Geometry check sheet. Reference: the model listing, model coordinates, mm. Round coordinates to 2 decimals unless told otherwise and drop trailing zeros. Order: outer loops, then holes, each group sorted by start corner. A loop starts at its lowest first (then second) coordinate and runs counter-clockwise, first axis right, second up. Notation, with made-up numbers: (89.25, 45.5) - (129.25, 45.5) arc R29 ccw to (129.25, 70.5) - close; hole circle Ø5 at (33.5, 35). An arc over 180 degrees is marked (long way). Answer as CSV lines item,"result". Start each with the question number.
```python
from build123d import *

# Parameters (mm, degrees)
SKETCH1_W           = 228.6
SKETCH1_H           = 457.2
BOSS_EXTRUDE1_DEPTH = 6.35
SKETCH2_W           = 6.35
SKETCH2_H           = 76.2
BOSS_EXTRUDE4_DEPTH = 6.35
SKETCH3_W           = 76.2
SKETCH3_H           = 6.35
CUT_EXTRUDE1_DEPTH  = 6.35


with BuildPart() as part:
    # Sketch1 → Boss-Extrude1 (new body)
    with BuildSketch(Plane.XY):
        with Locations((-78.307659574, -48.638297872)):
            Rectangle(SKETCH1_W, SKETCH1_H)
    extrude(amount=BOSS_EXTRUDE1_DEPTH)

    # Sketch2 → Boss-Extrude4 (add, through all)
    with BuildSketch(Plane.XY.offset(6.35)):
        with Locations((-195.782659574, 59.311702128)):
            Rectangle(SKETCH2_W, SKETCH2_H)
        with Locations((-195.782659574, -156.588297872)):
            Rectangle(SKETCH2_W, SKETCH2_H)
        with Locations((39.167340426, -156.588297872)):
            Rectangle(SKETCH2_W, SKETCH2_H)
        with Locations((39.167340426, 59.311702128)):
            Rectangle(SKETCH2_W, SKETCH2_H)
    extrude(amount=-BOSS_EXTRUDE4_DEPTH)

    # Sketch3 → Cut-Extrude1 (cut)
    with BuildSketch(Plane.XY.offset(6.35)):
        with Locations((-129.107659574, -274.063297872)):
            Rectangle(SKETCH3_W, SKETCH3_H)
        with Locations((-27.507659574, -274.063297872)):
            Rectangle(SKETCH3_W, SKETCH3_H)
        with Locations((-78.307659574, 176.786702128)):
            Rectangle(SKETCH3_W, SKETCH3_H)
    extrude(amount=-CUT_EXTRUDE1_DEPTH, mode=Mode.SUBTRACT)


solid = part.part
```
1. Thickness scan on probe 1 along Y at (x, z) = (-115, 2.5); probe 2 along X at (y, z) = (-20, 0.75); probe 3 along Y at (x, z) = (-128, 4.5). Record the ranges inside material, lowest first.
2. Section check B-B on y = -51.5. Record the boundary of the cut face in (x, z), plus the area to 3 significant figures.
3. Go/stop test with flat-tipped pins: pin 1 Ø3 at (y, z) = (-47, 2) entering from +X; pin 2 Ø3 at (x, z) = (-92, 4) entering from +Y; pin 3 Ø3 at (x, z) = (-114.5, 4.5) entering from -Y. Record where each tip stops, or that it passes through.
4. Section check C-C on x = -49.5. Record the boundary of the cut face in (y, z).
Numbers:
1,probe 1,"y = -270.89 to 173.61"
1,probe 2,"x = -192.61 to 35.99"
1,probe 3,"y = -270.89 to 179.96"
2,outline,"(-192.61, 0) - (35.99, 0) - (35.99, 6.35) - (-192.61, 6.35) - close"
2,area,"1,450 mm2"
3,pin 1,"stops at x = 35.99"
3,pin 2,"stops at y = 173.61"
3,pin 3,"stops at y = -270.89"
4,outline,"(-270.89, 0) - (173.61, 0) - (173.61, 6.35) - (-270.89, 6.35) - close"
